```python
from build123d import *

# Parameters (mm, degrees)
F0_W     = 2240
F0_H     = 1800
F1_DEPTH = 200
F2_W     = 1680
F2_H     = 1800
F3_DEPTH = 200
F4_W     = 1120
F4_H     = 1800
F5_DEPTH = 200
F6_W     = 560
F6_H     = 1800
F7_DEPTH = 200
F9_DEPTH = 1120


with BuildPart() as f1:
    # F0 (on Top) → F1 (new body)
    with BuildSketch(Plane.XY):
        Rectangle(F0_W, F0_H)
    extrude(amount=F1_DEPTH)

    # F2 (on face) → F3 (join)
    with BuildSketch(Plane.XY.offset(200)):
        with Locations((-280, 0)):
            Rectangle(F2_W, F2_H)
    extrude(amount=F3_DEPTH)

    # F4 (on face) → F5 (join)
    with BuildSketch(Plane.XY.offset(400)):
        with Locations((-560, 0)):
            Rectangle(F4_W, F4_H)
    extrude(amount=F5_DEPTH)

    # F6 (on face) → F7 (join)
    with BuildSketch(Plane.XY.offset(600)):
        with Locations((-840, 0)):
            Rectangle(F6_W, F6_H)
    extrude(amount=F7_DEPTH)

    # F8 (on face) → F9 (cut)
    with BuildSketch(Plane.YZ):
        with BuildLine():
            ThreePointArc((65, 500), (45.961941, 545.961941), (0, 565))
            Line((0, 565), (0, 500))
            Line((0, 500), (65, 500))
        make_face()
        with BuildLine():
            Line((0, 500), (0, 565))
            ThreePointArc((0, 565), (-45.961941, 454.038059), (65, 500))
            Line((65, 500), (0, 500))
        make_face()
    extrude(amount=-F9_DEPTH, mode=Mode.SUBTRACT)


solid = f1.part
```
Verification items for the finished model (mm, model axes). A direction names the side the tool comes from. Round coordinates to 2 decimals unless told otherwise and drop trailing zeros. Write each loop counter-clockwise with the first axis right and the second up, starting at its lowest first coordinate (ties: lowest second). Pieces come first, ordered by that corner, then holes. Notation, with made-up numbers: (-24, 21.25) -> (-10, 21.25) arc R21 cw to (-10, 42.25) -> close; hole circle Ø3 at (81, 50). An arc over 180 degrees is marked (long way). Write each question's results on one line, items separated by ' | '. Start each with the question number.
1. Cross-section at C-C (z = 675). Enter the section's corners in (x, y).
2. Cross-section at B-B (x = -369). Enter the section's corners in (y, z), then the cut area to 3 significant figures.
3. Set-up check for faces 1 (the flat face through (-284, 13, 600)), 2 (the flat face through (-844, 13, 800)): record each of +Z, -Z, +X, -X, +Y, -Y from which the full face is reachable in a straight line by a thin tool's end or side.
4. Cross-section at A-A (y = -297). Enter the section's corners in (x, z), then the cut area to 3 significant figures.
5. Cross-section at D-D (x = 658). Enter the section's corners in (y, z), then the cut area to 3 significant figures.
6. Material ranges on probe 1 along Y at (x, z) = (-444, 500); probe 2 along X at (y, z) = (681, 334); probe 3 along X at (y, z) = (386.5, 403), recorded low to high. Write a range as from..to.
7. Depth check by flat-ended pin: P1, Ø4, axis at y = 286.5, z = 275, coming from the +X side; P2, Ø5, axis at x = 202, y = 445, coming from the +Z side; P3, Ø3, axis at x = 24.5, y = -399, coming from the -Z side. Enter the tip coordinate at first touch or a pass-through.
Solutions:
1) outline: (-1120, -900) -> (-560, -900) -> (-560, 900) -> (-1120, 900) -> close
2) outline: (-900, 0) -> (900, 0) -> (900, 600) -> (-900, 600) -> close; hole circle Ø130 at (0, 500) | area: 1,070,000 mm2
3) face 1: +Z, +X, +Y, -Y | face 2: +Z, +X, -X, +Y, -Y
4) outline: (-1120, 0) -> (1120, 0) -> (1120, 200) -> (560, 200) -> (560, 400) -> (0, 400) -> (0, 600) -> (-560, 600) -> (-560, 800) -> (-1120, 800) -> close | area: 1,120,000 mm2
5) outline: (-900, 0) -> (900, 0) -> (900, 200) -> (-900, 200) -> close | area: 360,000 mm2
6) probe 1: y = -900..-65, 65..900 | probe 2: x = -1120..560 | probe 3: x = -1120..0
7) P1: stops at x = 560 | P2: stops at z = 400 | P3: stops at z = 0
